Geometry check sheet. Reference: the model listing, model coordinates, mm. A direction names the side the tool comes from. Give positions to 0.01 mm unless a question says otherwise; leave off trailing zeros. Write each loop counter-clockwise with the first axis right and the second up, starting at its lowest first coordinate (ties: lowest second). Pieces come first, ordered by that corner, then holes. Notation, with made-up numbers: (-17, 54.25) - (-1, 54.25) arc R28 cw to (-1, 72.25) - close; hole circle Ø6 at (-23.75, -16.5). An arc over 180 degrees is marked (long way). Write item = value, one per line. Start each with the question number.
(1) Section check B-B, the plane y = -18. Enter the section's corners in (x, z).
(2) Access from +Z, -Z, +X, -X, +Y, -Y to the whole of each face (thin tool, end or side, straight path). Record for faces 1 (the cylindrical face through (-3.434, 1.409, -0.776)), 2 (the flat face through (0, 0, 19.202)).
(3) Section check A-A, the plane x = 0. Enter the section's corners in (y, z), plus the area to 3 significant figures.
(4) Section check D-D, the plane x = -9.5. Enter the section's corners in (y, z), plus the area to 3 significant figures.
(5) Thickness scan on L1, parallel to Y at x = 0, z = 0.3; L2, parallel to Z at x = -11.5, y = -5; L3, parallel to Y at x = -3.5, z = 17. Record the ranges inside material, lowest first.
(6) Section check C-C, the plane z = 1.75. Enter the section's corners in (x, y), plus the area to 3 significant figures.
(7) Draft check along Y on faces 3 (the cylindrical face through (-5.483, 0.99, -5.682)), 4 (the cylindrical face through (0.261, 15.587, 0.369)), 5 (the flat face through (-2, -16, 0.749)), 6 (the cylindrical face through (0.261, -19.516, 0.369)). Enter one of: pulls with the +Y half, pulls with the -Y half, needs draft (parallel to the pull), parting line crosses it, or undercut.
(8) Depth check by flat-ended pin: pin 1 Ø8.5 at (x, y) = (-1, -6) entering from -Z; pin 2 Ø5.5 at (x, y) = (-0.5, 18) entering from +Z; pin 3 Ø0.8 at (y, z) = (-16, 0.5) entering from -X; pin 4 Ø8 at (x, z) = (0.5, 4) entering from -Y. Enter the tip coordinate at first touch or a pass-through.
```python
from build123d import *

# Parameters (mm, degrees)
BOSS_EXTRUDE1_DEPTH = 19.2024
SKETCH1_3_R         = 2.0066
BOSS_EXTRUDE2_DEPTH = 0.7493
SKETCH2_R           = 4.5212
BOSS_EXTRUDE3_DEPTH = 1.5748
SKETCH3_R           = 2.4511
BOSS_EXTRUDE4_DEPTH = 8.3312


with BuildPart() as part:
    # Sketch1 → Boss-Extrude1 (new body)
    with BuildSketch(Plane.XY):
        with BuildLine():
            Line((-3.5306, -13.516499682), (-3.5306, 13.516499682))
            ThreePointArc((-3.5306, 13.516499682), (-13.97, 0), (-3.5306, -13.516499682))
        make_face()
        with BuildLine():
            ThreePointArc((3.5052, 13.52310885), (-0.013122891, 13.969993836), (-3.5306, 13.516499682))
            Line((-3.5306, 13.516499682), (-3.5306, -13.516499682))
            ThreePointArc((-3.5306, -13.516499682), (-0.013122891, -13.969993836), (3.5052, -13.52310885))
            Line((3.5052, -13.52310885), (3.5052, 13.52310885))
        make_face()
        with BuildLine():
            ThreePointArc((13.97, 0), (11.048270091, 8.549656601), (3.5052, 13.52310885))
            Line((3.5052, 13.52310885), (3.5052, -13.52310885))
            ThreePointArc((3.5052, -13.52310885), (11.048270091, -8.549656601), (13.97, 0))
        make_face()
    extrude(amount=BOSS_EXTRUDE1_DEPTH)

    # Sketch1_3 → Boss-Extrude2 (add)
    # profile 1 of 2: a face of its own
    with BuildSketch(Plane.XY):
        with BuildLine():
            Line((3.5052, 13.52310885), (3.5052, 17.154059749))
            ThreePointArc((3.5052, 17.154059749), (0.211751316, 21.101044279), (-3.5306, 17.5768))
            Line((-3.5306, 17.5768), (-3.5306, 13.516499682))
            ThreePointArc((-3.5306, 13.516499682), (-0.013122891, 13.969993836), (3.5052, 13.52310885))
        make_face()
        with Locations(Location((0, 17.5768, 0), (0, 0, 180))):
            Circle(SKETCH1_3_R, mode=Mode.SUBTRACT)
    # profile 2 of 2: a face of its own
    with BuildSketch(Plane.XY):
        with BuildLine():
            ThreePointArc((3.5052, -13.52310885), (-0.013122891, -13.969993836), (-3.5306, -13.516499682))
            Line((-3.5306, -13.516499682), (-3.5306, -17.526))
            ThreePointArc((-3.5306, -17.526), (0.211751316, -21.050244279), (3.5052, -17.103259749))
            Line((3.5052, -17.103259749), (3.5052, -13.52310885))
        make_face()
        with Locations(Location((0, -17.526, 0), (0, 0, 180))):
            Circle(SKETCH1_3_R, mode=Mode.SUBTRACT)
    extrude(amount=BOSS_EXTRUDE2_DEPTH)

    # Sketch2 → Boss-Extrude3 (add)
    with BuildSketch(Plane.XY):
        with Locations((-7.746833441, 0.0508)):
            Circle(SKETCH2_R)
    extrude(amount=-BOSS_EXTRUDE3_DEPTH)

    # Sketch3 → Boss-Extrude4 (add)
    with BuildSketch(Plane(origin=(0, 0, -1.5748), x_dir=(-1, 0, 0), z_dir=(0, 0, -1))):
        with Locations(Location((7.746833441, 0.0508, 0), (0, 0, 180))):
            Circle(SKETCH3_R)
    extrude(amount=BOSS_EXTRUDE4_DEPTH)


solid = part.part
```
Model answer:
q1.outline = (-3.5, 0) - (-1.95, 0) - (-1.95, 0.75) - (-3.5, 0.75) - close; (1.95, 0) - (3.5, 0) - (3.5, 0.75) - (1.95, 0.75) - close
q2.face_1 = -Z
q2.face_2 = +Z, +X, -X, +Y, -Y
q3.outline = (-21.06, 0) - (-19.53, 0) - (-19.53, 0.75) - (-21.06, 0.75) - close; (-15.52, 0) - (15.57, 0) - (15.57, 0.75) - (13.97, 0.75) - (13.97, 19.2) - (-13.97, 19.2) - (-13.97, 0.75) - (-15.52, 0.75) - close; (19.58, 0) - (21.11, 0) - (21.11, 0.75) - (19.58, 0.75) - close
q3.area = 541 mm²
q4.outline = (-10.24, 0) - (-4.12, 0) - (-4.12, -1.57) - (-1.66, -1.57) - (-1.66, -9.91) - (1.76, -9.91) - (1.76, -1.57) - (4.22, -1.57) - (4.22, 0) - (10.24, 0) - (10.24, 19.2) - (-10.24, 19.2) - close
q4.area = 435 mm²
q5.L1 = -21.06 to -19.53, -15.52 to 15.57, 19.58 to 21.11
q5.L2 = 0 to 19.2
q5.L3 = -13.52 to 13.52
q6.outline = circle Ø27.94 at (0, 0)
q6.area = 613 mm²
q7.face_3 = parting line crosses it
q7.face_4 = undercut
q7.face_5 = needs draft
q7.face_6 = undercut
q8.pin_1 = 0
q8.pin_2 = 0.75
q8.pin_3 = -3.53
q8.pin_4 = -21.06
